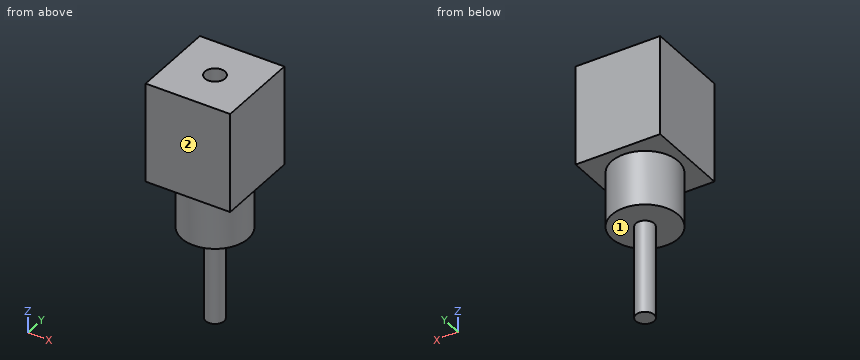
```python
from build123d import *

# Parameters (mm, degrees)
SKETCH1_W           = 2.54
SKETCH1_H           = 2.54
BOSS_EXTRUDE1_DEPTH = 3
SKETCH2_R           = 1
BOSS_EXTRUDE2_DEPTH = 1.64
SKETCH3_R           = 0.275
BOSS_EXTRUDE3_DEPTH = 2.79
SKETCH4_R           = 0.3
CUT_EXTRUDE1_DEPTH  = 3


with BuildPart() as part:
    # Sketch1 → Boss-Extrude1 (new body)
    with BuildSketch(Plane.XY):
        Rectangle(SKETCH1_W, SKETCH1_H)
    extrude(amount=BOSS_EXTRUDE1_DEPTH)

    # Sketch2 → Boss-Extrude2 (add)
    with BuildSketch(Plane(origin=(0, 0, 0), x_dir=(-1, 0, 0), z_dir=(0, 0, -1))):
        Circle(SKETCH2_R)
    extrude(amount=BOSS_EXTRUDE2_DEPTH)

    # Sketch3 → Boss-Extrude3 (add)
    with BuildSketch(Plane(origin=(0, 0, -1.64), x_dir=(-1, 0, 0), z_dir=(0, 0, -1))):
        Circle(SKETCH3_R)
    extrude(amount=BOSS_EXTRUDE3_DEPTH)

    # Sketch4 → Cut-Extrude1 (cut)
    with BuildSketch(Plane.XY.offset(3)):
        Circle(SKETCH4_R)
    extrude(amount=-CUT_EXTRUDE1_DEPTH, mode=Mode.SUBTRACT)


solid = part.part
```
The model under review builds one solid part; all positions refer to its coordinate system, in mm. Face numbers are marked on the shaded views. A direction names the side the tool comes from. Round coordinates to 2 decimals unless told otherwise and drop trailing zeros. Order: outer loops, then holes, each group sorted by start corner. A loop starts at its lowest first (then second) coordinate and runs counter-clockwise, first axis right, second up. Notation, with made-up numbers: (7.25, 19) - (23.25, 19) arc R33 ccw to (23.25, 53) - close; hole circle Ø1 at (78.5, 81). An arc over 180 degrees is marked (long way). Answer in a Markdown table with one row per item.
(1) Take a section at D-D on z = -2.75. Write out the cut boundary in (x, y) (3 decimals).
Result set:
| item | result |
|---|---|
| outline | circle Ø0.55 at (0, 0) |
(2) Clearance check with flat-ended pins moving along their axes: P1, Ø0.5, axis at x = 0, y = 0, coming from the +Z side; P2, Ø1, axis at y = -0.5, z = -2, coming from the -X side. State where each tip first meets the part, or that it passes through.
Result set:
| item | result |
|---|---|
| P1 | stops at z = 0 |
| P2 | stops at x = -0.99 |
(3) Take a section at B-B on x = 0. Write out the cut boundary in (y, z) (3 decimals), plus the area to 3 significant figures.
Result set:
| item | result |
|---|---|
| outline | (-1.27, 0) - (-1, 0) - (-1, -1.64) - (-0.275, -1.64) - (-0.275, -4.43) - (0.275, -4.43) - (0.275, -1.64) - (1, -1.64) - (1, 0) - (1.27, 0) - (1.27, 3) - (0.3, 3) - (0.3, 0) - (-0.3, 0) - (-0.3, 3) - (-1.27, 3) - close |
| area | 10.6 mm2 |
(4) Machinability: for the marked faces 1 and 2, which of the approach directions +Z, -Z, +X, -X, +Y, -Y give a long, thin tool a straight path to every point of the face, cutting with its end or side? Answer none if there is none.
Result set:
| item | result |
|---|---|
| face 1 | -Z |
| face 2 | +Z, -Z, +X, -X, -Y |
(5) Take a section at C-C on z = 1.5. Write out the cut boundary in (x, y), plus the area to 3 significant figures.
Result set:
| item | result |
|---|---|
| outline | (-1.27, -1.27) - (1.27, -1.27) - (1.27, 1.27) - (-1.27, 1.27) - close; hole circle Ø0.6 at (0, 0) |
| area | 6.17 mm2 |
(6) Take a section at A-A on y = -0.6. Write out the cut boundary in (x, z), plus the area to 3 significant figures.
Result set:
| item | result |
|---|---|
| outline | (-1.27, 0) - (-0.8, 0) - (-0.8, -1.64) - (0.8, -1.64) - (0.8, 0) - (1.27, 0) - (1.27, 3) - (-1.27, 3) - close |
| area | 10.2 mm2 |
(7) For line 1 (Y direction, x = 0, z = 0.8); line 2 (Z direction, x = -0.95, y = -0.4); line 3 (Z direction, x = -0.8, y = 0.3), list the stretches that pass through material, from the lowest coordinate up. Write a range as from..to.
Result set:
| item | result |
|---|---|
| line 1 | y = -1.27..-0.3, 0.3..1.27 |
| line 2 | z = 0..3 |
| line 3 | z = -1.64..3 |
